from build123d import *

# Parameters (mm, degrees)
SKETCH1_R               = 3.3782
BOSS_EXTRUDE1_DEPTH     = 11.1125
SKETCH2_R               = 3.3655
CUT_EXTRUDE1_DEPTH      = 422.26425461
SKETCH3_R               = 3.3655
CUT_EXTRUDE2_DEPTH      = 422.154164722
SKETCH4_R               = 3.3655
CUT_EXTRUDE3_DEPTH      = 422.154164722
SKETCH5_R               = 3.3655
CUT_EXTRUDE4_DEPTH      = 422.154164722
CUT_EXTRUDE5_DEPTH      = 422.369531068
CUT_EXTRUDE5_DEPTH_BACK = 422.369531068
SKETCH6_R               = 3.3782
SKETCH7_W               = 19.45
SKETCH7_H               = 169.071428571
CUT_EXTRUDE6_DEPTH      = 694.733868394
BOSS_EXTRUDE2_DEPTH     = 11.1125


with BuildPart() as part:
    # Sketch1 → Boss-Extrude1 (new body)
    with BuildSketch(Plane.XY):
        Polygon((-629.05, -12.5), (-568.725, -12.5), (-568.725, 76.762), (-74.813700004, 76.762), (-74.813700004, -12.5), (0, -12.5), (0, 216.1), (-63.5, 292.3), (-451.25, 292.3), (-629.05, 139.9), align=None)
        with Locations((-12.5, 203.6)):
            Circle(SKETCH1_R, mode=Mode.SUBTRACT)
        with BuildLine():
            Line((-460.428573591, 202.287851535), (-452.336342065, 200.199533722))
            ThreePointArc((-452.336342065, 200.199533722), (-451.339589022, 199.42298326), (-451.225592299, 198.164590635))
            Line((-451.225592299, 198.164590635), (-451.993143659, 195.840315389))
            ThreePointArc((-451.993143659, 195.840315389), (-452.739984992, 194.944683826), (-453.897256136, 194.800977973))
            Line((-453.897256136, 194.800977973), (-461.832222689, 196.848711278))
            ThreePointArc((-461.832222689, 196.848711278), (-462.802959706, 197.57942531), (-462.972681585, 198.782532884))
            Line((-462.972681585, 198.782532884), (-462.362395197, 201.147392639))
            ThreePointArc((-462.362395197, 201.147392639), (-461.631681165, 202.118129655), (-460.428573591, 202.287851535))
        make_face(mode=Mode.SUBTRACT)
    extrude(amount=BOSS_EXTRUDE1_DEPTH)

    # Sketch2 → Cut-Extrude1 (cut, through all)
    with BuildSketch(Plane(origin=(-305, 23.6125, -5.08), x_dir=(-1, 0, 0), z_dir=(0, 0, -1))):
        with Locations((288.9533823, 103.7145)):
            Circle(SKETCH2_R)
    extrude(amount=-CUT_EXTRUDE1_DEPTH, mode=Mode.SUBTRACT)

    # Sketch3 → Cut-Extrude2 (cut, through all)
    with BuildSketch(Plane(origin=(-305, 23.6125, -1.905), x_dir=(-1, 0, 0), z_dir=(0, 0, -1))):
        with Locations((143.116254523, 256.904809604)):
            Circle(SKETCH3_R)
    extrude(amount=-CUT_EXTRUDE2_DEPTH, mode=Mode.SUBTRACT)

    # Sketch4 → Cut-Extrude3 (cut, through all)
    with BuildSketch(Plane(origin=(-305, 23.6125, -1.905), x_dir=(-1, 0, 0), z_dir=(0, 0, -1))):
        with Locations((-47.625, 250.9075)):
            Circle(SKETCH4_R)
    extrude(amount=-CUT_EXTRUDE3_DEPTH, mode=Mode.SUBTRACT)

    # Sketch5 → Cut-Extrude4 (cut, through all)
    with BuildSketch(Plane(origin=(-305, 23.6125, -1.905), x_dir=(-1, 0, 0), z_dir=(0, 0, -1))):
        with Locations((-236.766660116, 257.207608298)):
            Circle(SKETCH5_R)
    extrude(amount=-CUT_EXTRUDE4_DEPTH, mode=Mode.SUBTRACT)

    # Sketch6 → Cut-Extrude5 (cut, two sides: drawn at the far end of the back side and taken through both)
    with BuildSketch(Plane(origin=(-305, 23.6125, 18.7325), x_dir=(1, 0, 0), z_dir=(0, 0, 1)).offset(-CUT_EXTRUDE5_DEPTH_BACK)):
        with Locations((-197.262125611, 186.926969688)):
            Circle(SKETCH6_R)
        with Locations((-33.209654284, 70.005387803)):
            Circle(SKETCH6_R)
        with Locations((-90.296950895, 152.235012548)):
            Circle(SKETCH6_R)
    extrude(amount=CUT_EXTRUDE5_DEPTH + CUT_EXTRUDE5_DEPTH_BACK, mode=Mode.SUBTRACT)

    # Sketch7 → Cut-Extrude6 (cut, through all)
    with BuildSketch(Plane.XY.offset(11.1125)):
        with Locations((-619.325, 72.035714286)):
            Rectangle(SKETCH7_W, SKETCH7_H)
    extrude(amount=-CUT_EXTRUDE6_DEPTH, mode=Mode.SUBTRACT)

    # Sketch9 → Boss-Extrude2 (add)
    with BuildSketch(Plane.XY.offset(11.1125)):
        Polygon((0, 216.1), (0, 245.857051265), (-24.6799078, 275.472940625), (-39.314523176, 263.277427812), align=None)
    extrude(amount=-BOSS_EXTRUDE2_DEPTH)


solid = part.part
Source: CAD feature listing. Evaluate the final solid. Frame: model axes, mm. A direction names the side the tool comes from. Give positions to 0.01 mm unless a question says otherwise; leave off trailing zeros. Order: outer loops, then holes, each group sorted by start corner. A loop starts at its lowest first (then second) coordinate and runs counter-clockwise, first axis right, second up. Notation, with made-up numbers: (35.25, -6.75) -> (42.25, -6.75) arc R19 ccw to (42.25, 24.25) -> close; hole circle Ø10 at (44.25, 57). An arc over 180 degrees is marked (long way). Write item = value, one per line.
Item 1: Ray query, probe 1 along X at (y, z) = (32.5, 8) (3 decimals); probe 2 along X at (y, z) = (273, 2.25); probe 3 along X at (y, z) = (279, 8.5). Return the intervals inside material, ascending.
Check result:
probe_1 = -609.6 to -568.725, -74.814 to 0
probe_2 = -473.77 to -260.38, -254.37 to -47.42, -27.65 to -22.62
probe_3 = -466.77 to -451.12, -445.11 to -71.06, -65.4 to -52.42
Item 2: Set-up query: faces 1 (the face through (-31.895, 269.461, 5.634)), 2 (the face through (-529.3, 225.4, 5.5)), 3 (the face through (-74.814, 33, 5)). Return all of +Z, -Z, +X, -X, +Y, -Y with unobstructed straight access to the full face (end or side cutting, diameter ignored); none if empty.
Check result:
face_1 = +Z, -Z, +Y
face_2 = +Z, -Z, -X, +Y
face_3 = +Z, -Z, -Y
Item 3: Section query A-A (z = 9.25). State how many separate pieces and enclosed holes the cut face has, then the cut area to 3 significant figures.
Check result:
separate_pieces = 1
enclosed_holes = 9
area = 129,000 mm²
Item 4: Section query B-B (x = -326.5). Output: boundary loops of the cut face in (y, z).
Check result:
outline = (76.76, 0) -> (292.3, 0) -> (292.3, 11.11) -> (76.76, 11.11) -> close
Item 5: Contact query for a flat-ended pin moving along its axis: pin 1 (5 mm diameter, centred on y = 254.5, z = 9, fed in from +X). Output: stop coordinate, or through.
Check result:
pin_1 = -5.12
Item 6: Mould query, pull axis X, two halves, no side actions, for faces 4 (the face through (-589, -12.5, 5)), 5 (the face through (-609.6, 71, 6)), 6 (the face through (-325, 76.762, 5)). Classes: +X half, -X half, draft (parallel to the pull), parting line (faces both ways), or undercut.
Check result:
face_4 = draft
face_5 = -X half
face_6 = undercut
